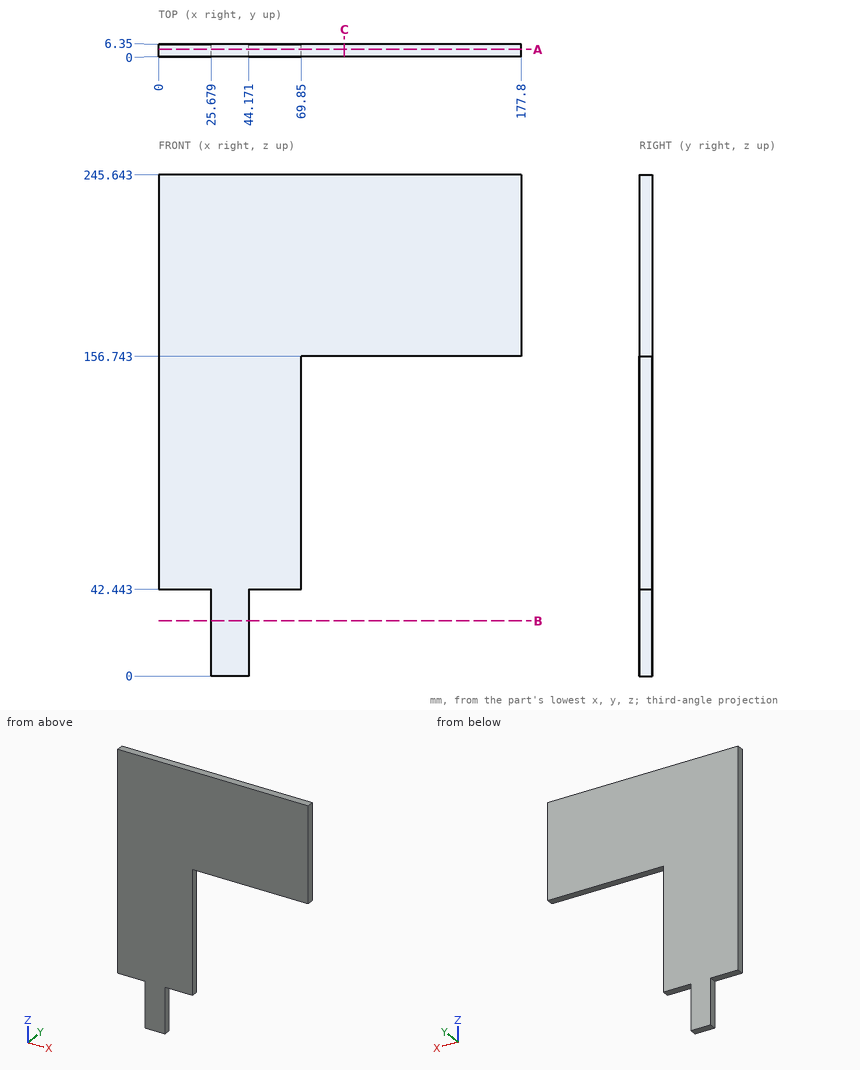
Answer from the drawing. Dimensions are ordinates in mm from the lowest x, y and z of the part. Round coordinates to 2 decimals unless told otherwise and drop trailing zeros. Write each loop counter-clockwise with the first axis right and the second up, starting at its lowest first coordinate (ties: lowest second). Pieces come first, ordered by that corner, then holes. Notation, with made-up numbers: (72, 47.25) - (110, 47.25) arc R11 cw to (110, 56.25) - close; hole circle Ø11 at (-9.75, 11.25). An arc over 180 degrees is marked (long way). One line per item, written item: value.
Q1. Straight lines are drawn through the part: line 1 (Z direction, x = 167.5, y = 3.75); line 2 (X direction, y = 5.5, z = 132); line 3 (Z direction, x = 8.5, y = 3.75). For each, find the intervals that lie inside material, in ascending order. Write a range as from..to.
The answers:
line 1: z = 156.74..245.64
line 2: x = 0..69.85
line 3: z = 42.44..245.64
Q2. Find section A-A (y = 3.75). Determine the outline of the cut face in (x, z), and give its area (3 significant figures).
The answers:
outline: (0, 42.44) - (25.68, 42.44) - (25.68, 0) - (44.17, 0) - (44.17, 42.44) - (69.85, 42.44) - (69.85, 156.74) - (177.8, 156.74) - (177.8, 245.64) - (0, 245.64) - close
area: 24,600 mm2
Q3. Find section B-B (z = 27). Determine the outline of the cut face in (x, y), and give its area (3 significant figures).
The answers:
outline: (25.68, 0) - (44.17, 0) - (44.17, 6.35) - (25.68, 6.35) - close
area: 117 mm2
Q4. Each of these flat-tipped pins is pushed along its axis until it touches: P1, Ø1.9, axis at x = 123.5, y = 2.5, coming from the -Z side; P2, Ø1.9, axis at x = 51.5, y = 4, coming from the -Z side; P3, Ø3, axis at y = 4.5, z = 26.5, coming from the -X side. Where does it stop, or does it pass through?
The answers:
P1: stops at z = 156.74
P2: stops at z = 42.44
P3: stops at x = 25.68
Q5. Find section C-C (x = 91). Determine the outline of the cut face in (y, z).
The answers:
outline: (0, 156.74) - (6.35, 156.74) - (6.35, 245.64) - (0, 245.64) - close
